```python
from build123d import *

# Parameters (mm, degrees)
SKETCH2_W           = 105
SKETCH2_H           = 110
BOSS_EXTRUDE1_DEPTH = 2
SKETCH4_W           = 18
SKETCH4_H           = 2
SKETCH4_W_2         = 105
BOSS_EXTRUDE2_DEPTH = 20


with BuildPart() as part:
    # Sketch2 → Boss-Extrude1 (new body)
    with BuildSketch(Plane(origin=(0, 0, 0), x_dir=(1, 0, 0), z_dir=(0, 1, 0))):
        Rectangle(SKETCH2_W, SKETCH2_H)
    extrude(amount=BOSS_EXTRUDE1_DEPTH)

    # Sketch4 → Boss-Extrude2 (add)
    with BuildSketch(Plane(origin=(0, 2, 0), x_dir=(1, 0, 0), z_dir=(0, 1, 0))):
        with Locations((-43.5, 26.895070822)):
            Rectangle(SKETCH4_W, SKETCH4_H)
        with Locations((-43.5, 8.934071448)):
            Rectangle(SKETCH4_W, SKETCH4_H)
        with Locations((-43.5, -9.04022418)):
            Rectangle(SKETCH4_W, SKETCH4_H)
        with Locations((-43.5, -27.006397159)):
            Rectangle(SKETCH4_W, SKETCH4_H)
        with Locations((0, 54)):
            Rectangle(SKETCH4_W_2, SKETCH4_H)
        with Locations((0, -54)):
            Rectangle(SKETCH4_W_2, SKETCH4_H)
    extrude(amount=BOSS_EXTRUDE2_DEPTH)


solid = part.part
```
Could you check a few things on this model? Use its own coordinates, in mm. A direction names the side the tool comes from. Coordinates: 2 decimals unless noted, no trailing zeros. Write each loop counter-clockwise with the first axis right and the second up, starting at its lowest first coordinate (ties: lowest second). Pieces come first, ordered by that corner, then holes. Notation, with made-up numbers: (68, -33) - (86, -33) arc R19 cw to (86, -18) - close; hole circle Ø1 at (86, 80.5). An arc over 180 degrees is marked (long way). Use a Markdown table: item, result.
Q1. Imagine slicing it at B-B (x = 28). List the corners of the cut face in (y, z) for me.
Geometry check:
| item | result |
|---|---|
| outline | (0, -55) - (22, -55) - (22, -53) - (2, -53) - (2, 53) - (22, 53) - (22, 55) - (0, 55) - close |
Q2. Imagine slicing it at C-C (z = 33). List the corners of the cut face in (x, y) for me, and give its area (3 significant figures).
Geometry check:
| item | result |
|---|---|
| outline | (-52.5, 0) - (52.5, 0) - (52.5, 2) - (-52.5, 2) - close |
| area | 210 mm2 |
Q3. Please list where these lines run through material, in increasing order: L1, parallel to Z at x = -35.5, y = 20.5; L2, parallel to Z at x = 23, y = 11; L3, parallel to Y at x = 0.5, z = 2.5.
Geometry check:
| item | result |
|---|---|
| L1 | z = -55 to -53, -27.9 to -25.9, -9.93 to -7.93, 8.04 to 10.04, 26.01 to 28.01, 53 to 55 |
| L2 | z = -55 to -53, 53 to 55 |
| L3 | y = 0 to 2 |
Q4. I'm going to push flat-ended pins straight in: pin 1 Ø8 at (x, z) = (-37, 36.5) entering from -Y; pin 2 Ø1.6 at (y, z) = (14.5, 9) entering from +X; pin 3 Ø3 at (x, z) = (7.5, 28.5) entering from +Y. Where does each tip first touch, or does it pass through?
Geometry check:
| item | result |
|---|---|
| pin 1 | stops at y = 0 |
| pin 2 | stops at x = -34.5 |
| pin 3 | stops at y = 2 |
Q5. Imagine slicing it at A-A (y = 16.5). List the corners of the cut face in (x, z) for me.
Geometry check:
| item | result |
|---|---|
| outline | (-52.5, -55) - (52.5, -55) - (52.5, -53) - (-52.5, -53) - close; (-52.5, -27.9) - (-34.5, -27.9) - (-34.5, -25.9) - (-52.5, -25.9) - close; (-52.5, -9.93) - (-34.5, -9.93) - (-34.5, -7.93) - (-52.5, -7.93) - close; (-52.5, 8.04) - (-34.5, 8.04) - (-34.5, 10.04) - (-52.5, 10.04) - close; (-52.5, 26.01) - (-34.5, 26.01) - (-34.5, 28.01) - (-52.5, 28.01) - close; (-52.5, 53) - (52.5, 53) - (52.5, 55) - (-52.5, 55) - close |
Q6. Thinking about a two-plate mould opening in Z: for faces 3 (the flat face through (-1, 2, -1)), 4 (the flat face through (-44, 12, 8.04)), 5 (the flat face through (-1, 11, 55)), 6 (the flat face through (-1, 11, -55)), which applies, +Z half, -Z half, draft (parallel to the pull), parting line (faces both ways), or undercut?
Geometry check:
| item | result |
|---|---|
| face 3 | undercut |
| face 4 | undercut |
| face 5 | +Z half |
| face 6 | -Z half |
Q7. Which directions (+Z, -Z, +X, -X, +Y, -Y) give clear straight access to the entire face, cutting with the end or side of a thin tool? Please do faces 1 (the flat face through (-1, 0, -1)), 2 (the flat face through (-1, 12, 53)).
Geometry check:
| item | result |
|---|---|
| face 1 | +Z, -Z, +X, -X, -Y |
| face 2 | +X, -X, +Y |
